Check sheet for the modelled part. Datum: model origin and axes. Units: mm. Face numbers are marked on the shaded views. A direction names the side the tool comes from. Round coordinates to 2 decimals unless told otherwise and drop trailing zeros. Write each loop counter-clockwise with the first axis right and the second up, starting at its lowest first coordinate (ties: lowest second). Pieces come first, ordered by that corner, then holes. Notation, with made-up numbers: (-35, -14) - (7, -14) arc R22 cw to (7, 16) - close; hole circle Ø10 at (-25, 31). An arc over 180 degrees is marked (long way). Answer as a JSON object with one key per item and string values. Group by question number.
Item 1: Gauge pin test, flat ends, axial feed: P1, Ø9.5, axis at x = -0.5, z = 9, coming from the -Y side; P2, Ø5.5, axis at x = -2.5, y = -6.5, coming from the -Z side; P3, Ø1, axis at x = 10.5, y = -8.5, coming from the +Z side. Record the tip position at first contact, or that the pin passes through.
Item 2: Thickness scan on line 1 (Z direction, x = 0, y = 0.4); line 2 (X direction, y = 0.35, z = 5.5); line 3 (Y direction, x = -13, z = 15.25). Record the ranges inside material, lowest first.
Item 3: Set-up check for the marked faces 1 and 2: record each of +Z, -Z, +X, -X, +Y, -Y from which the full face is reachable in a straight line by a thin tool's end or side.
Item 4: Release check for a two-part mould opening along X. For the marked faces 3, 4, 5 and 6 record: pulls with the +X half, pulls with the -X half, needs draft (parallel to the pull), parting line crosses it, or undercut.
Item 5: Sectioned sample at C-C on z = 5.5. Record the boundary of the cut face in (x, y).
Item 6: Sectioned sample at A-A on x = 0. Record the boundary of the cut face in (y, z) (3 decimals).
Item 7: Sectioned sample at D-D on x = -3.5. Record the boundary of the cut face in (y, z).
Item 8: Sectioned sample at B-B on y = -6. Record the boundary of the cut face in (x, z) (3 decimals).
```python
from build123d import *

# Parameters (mm, degrees)
BOSS_EXTRUDE1_DEPTH = 2
BOSS_EXTRUDE2_DEPTH = 13
CUT_EXTRUDE1_DEPTH  = 7


with BuildPart() as part:
    # Sketch1 → Boss-Extrude1 (new body)
    with BuildSketch(Plane(origin=(0, 0, 0), x_dir=(1, 0, 0), z_dir=(0, 1, 0))):
        Polygon((-15, -14.4), (-15, 0), (15, 0), (15, -14.4), (5.71590909, -18.700000004), (-5.71590909, -18.700000004), align=None)
    extrude(amount=BOSS_EXTRUDE1_DEPTH)

    # Sketch3 → CSK for M3 Flat Head Machine Screw1 (revolve, cut)
    with BuildSketch(Plane(origin=(0, 2, 5.5), x_dir=(0, 0, 1), z_dir=(1, 0, 0))):
        Polygon((0, 0), (0, 2), (1.7, 2), (1.7, 1.45), (3.15, 0), align=None)
    revolve(axis=Axis((0, 8.35, 5.5), (0, -1, 0)), mode=Mode.SUBTRACT)

    # Sketch4 → Boss-Extrude2 (add)
    with BuildSketch(Plane(origin=(0, 2, 0), x_dir=(1, 0, 0), z_dir=(0, 1, 0))):
        Polygon((-15, -14.4), (-15, -16.33369736), (-5.572755662, -20.700000004), (5.5, -20.700000004), (15, -16.3), (15, -14.4), (5.71590909, -18.700000004), (-5.71590909, -18.700000004), align=None)
    extrude(amount=-BOSS_EXTRUDE2_DEPTH)

    # Sketch5 → Cut-Extrude1 (cut)
    with BuildSketch(Plane.XY.offset(20.700000004)):
        with BuildLine():
            Line((1.825, -4.5), (1.825, -11))
            ThreePointArc((1.825, -11), (0, -12.825), (-1.825, -11))
            Line((-1.825, -11), (-1.825, -4.5))
            ThreePointArc((-1.825, -4.5), (0, -2.675), (1.825, -4.5))
        make_face()
    extrude(amount=-CUT_EXTRUDE1_DEPTH, mode=Mode.SUBTRACT)


solid = part.part
```
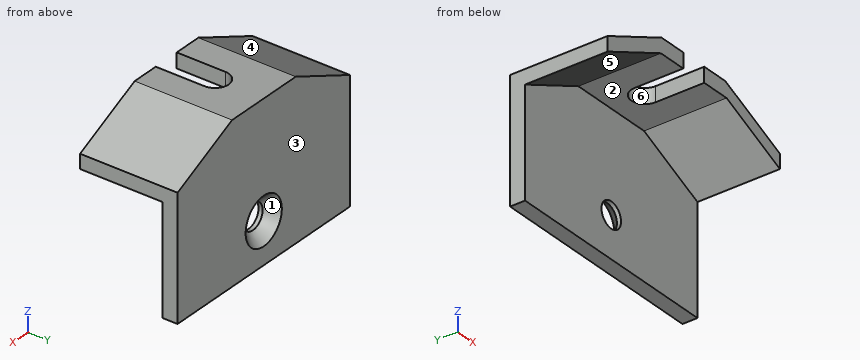
Completed:
{
 "1": {"P1": "y = 0", "P2": "z = 18.7", "P3": "z = 18.62"},
 "2": {"line 1": "0 to 3.8, 7.2 to 20.7", "line 2": "-15 to -1.7, 1.7 to 15", "line 3": "0 to 2"},
 "3": {"face 1": "+Y", "face 2": "-Z, -Y"},
 "4": {"face 3": "needs draft", "face 4": "pulls with the -X half", "face 5": "undercut", "face 6": "undercut"},
 "5": {"outline": "(-15, 0) - (-1.7, 0) - (-1.7, 0.55) - (-3.15, 2) - (-15, 2) - close; (1.7, 0) - (15, 0) - (15, 2) - (3.15, 2) - (1.7, 0.55) - close"},
 "6": {"outline": "(-2.675, 18.7) - (0, 18.7) - (0, 7.2) - (0.55, 7.2) - (2, 8.65) - (2, 20.7) - (-2.675, 20.7) - close; (0, 0) - (2, 0) - (2, 2.35) - (0.55, 3.8) - (0, 3.8) - close"},
 "7": {"outline": "(-11, 18.7) - (0, 18.7) - (0, 0) - (2, 0) - (2, 20.7) - (-11, 20.7) - close"},
 "8": {"outline": "(-15, 14.4) - (-5.716, 18.7) - (-1.825, 18.7) - (-1.825, 20.7) - (-5.573, 20.7) - (-15, 16.334) - close; (1.825, 18.7) - (5.716, 18.7) - (15, 14.4) - (15, 16.3) - (5.5, 20.7) - (1.825, 20.7) - close"}
}
